```python
from build123d import *

# Parameters (mm, degrees)
BOSS_EXTRUDE1_DEPTH = 10
SKETCH2_R           = 6
BOSS_EXTRUDE2_DEPTH = 10
SKETCH3_R           = 2.925
CUT_EXTRUDE1_DEPTH  = 21
FILLET1_R           = 4
CHAMFER1_SIZE       = 5


with BuildPart() as part:
    # Sketch1 → Boss-Extrude1 (new body)
    with BuildSketch(Plane(origin=(0, 0, 0), x_dir=(1, 0, 0), z_dir=(0, 1, 0))):
        Polygon((7.764943234, 13.989483785), (-8.232776727, 13.719379992), (-15.997719961, -0.270103793), (-7.764943234, -13.989483785), (8.232776727, -13.719379992), (15.997719961, 0.270103793), align=None)
    extrude(amount=BOSS_EXTRUDE1_DEPTH)

    # Sketch2 → Boss-Extrude2 (add)
    with BuildSketch(Plane.XZ):
        Circle(SKETCH2_R)
    extrude(amount=BOSS_EXTRUDE2_DEPTH)

    # Sketch3 → Cut-Extrude1 (cut, through all)
    with BuildSketch(Plane.XZ.offset(10)):
        Circle(SKETCH3_R)
    extrude(amount=-CUT_EXTRUDE1_DEPTH, mode=Mode.SUBTRACT)

    # Fillet1
    fillet1_edges = [part.edges().sort_by_distance(p)[0] for p in [
        (-6, 0, 0),
    ]]
    fillet(fillet1_edges, radius=FILLET1_R)

    # Chamfer1
    chamfer1_edges = [part.edges().sort_by_distance(p)[0] for p in [
        (-2.925, 10, 0),
    ]]
    chamfer(chamfer1_edges, length=CHAMFER1_SIZE)


solid = part.part
```
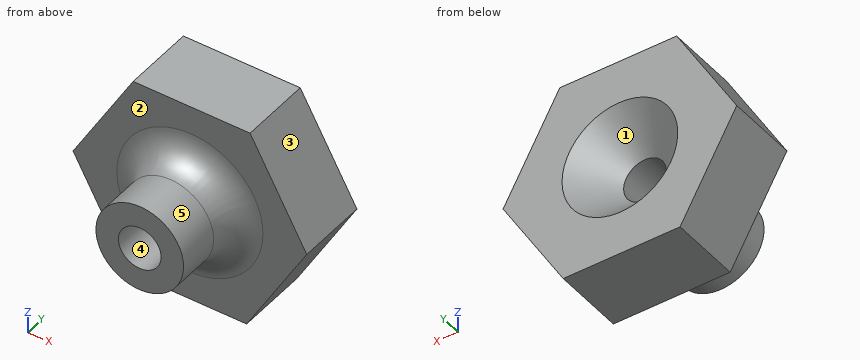
Geometry: final body of the model. Coordinates: model frame, mm. Face numbers are marked on the shaded views. A direction names the side the tool comes from. Coordinates: 2 decimals unless noted, no trailing zeros. Order: outer loops, then holes, each group sorted by start corner. A loop starts at its lowest first (then second) coordinate and runs counter-clockwise, first axis right, second up. Notation, with made-up numbers: (53.5, 43.5) - (104.5, 43.5) arc R22 cw to (104.5, 64.5) - close; hole circle Ø7 at (88, 86.5). An arc over 180 degrees is marked (long way). Write each question's results on one line, items separated by ' | '.
1) Pull-direction query (X, two-part tool) for the marked faces 3, 4 and 5; classes: pulls with the +X half, pulls with the -X half, needs draft (parallel to the pull), parting line crosses it, or undercut.
Results list:
face 3: pulls with the +X half | face 4: undercut | face 5: parting line crosses it
2) Section B-B, the plane x = 0. Return loops of the section in (y, z) (3 decimals), plus the area to 3 significant figures.
Results list:
outline: (-10, -6) - (-4, -6) arc R4 cw to (0, -10) - (0, -13.858) - (10, -13.858) - (10, -7.925) - (5, -2.925) - (-10, -2.925) - close; (-10, 2.925) - (5, 2.925) - (10, 7.925) - (10, 13.858) - (0, 13.858) - (0, 10) arc R4 cw to (-4, 6) - (-10, 6) - close | area: 262 mm^2
3) Set-up query: the marked faces 1 and 2. Return all of +Z, -Z, +X, -X, +Y, -Y with unobstructed straight access to the full face (end or side cutting, diameter ignored); none if empty.
Results list:
face 1: +Y | face 2: -Y
4) Section A-A, the plane y = 3.5. Return loops of the section in (x, z) (3 decimals).
Results list:
outline: (-15.998, 0.27) - (-8.233, -13.719) - (7.765, -13.989) - (15.998, -0.27) - (8.233, 13.719) - (-7.765, 13.989) - close; hole circle Ø5.85 at (0, 0)
5) Line query: line 1 (Z direction, x = 0, y = -5.25) (3 decimals); line 2 (Z direction, x = 0, y = -1.5) (1 decimal); line 3 (Y direction, x = -9, z = -9.25). Output: solid intervals per line, ascending. Write a range as from..to.
Results list:
line 1: -6..-2.925, 2.925..6 | line 2: -6.9..-2.9, 2.9..6.9 | line 3: 0..10
6) Pin query (flat end, axial travel): pin 1 (6.5 mm diameter, centred on x = 0, z = 0, fed in from +Y) (3 decimals); pin 2 (1 mm diameter, centred on y = -7, z = 5.5, fed in from -X); pin 3 (1.5 mm diameter, centred on x = -5, y = 2, fed in from -Z). Return the tip coordinate at first contact, or that it passes through.
Results list:
pin 1: y = 5.325 | pin 2: x = -3.32 | pin 3: z = -13.79
7) Section D-D, the plane x = -13. Return loops of the section in (y, z).
Results list:
outline: (0, -5.13) - (10, -5.13) - (10, 5.27) - (0, 5.27) - close
8) Section C-C, the plane y = -7. Return loops of the section in (x, z) (3 decimals), plus the area to 3 significant figures.
Results list:
outline: circle Ø12 at (0, 0); hole circle Ø5.85 at (0, 0) | area: 86.2 mm^2
